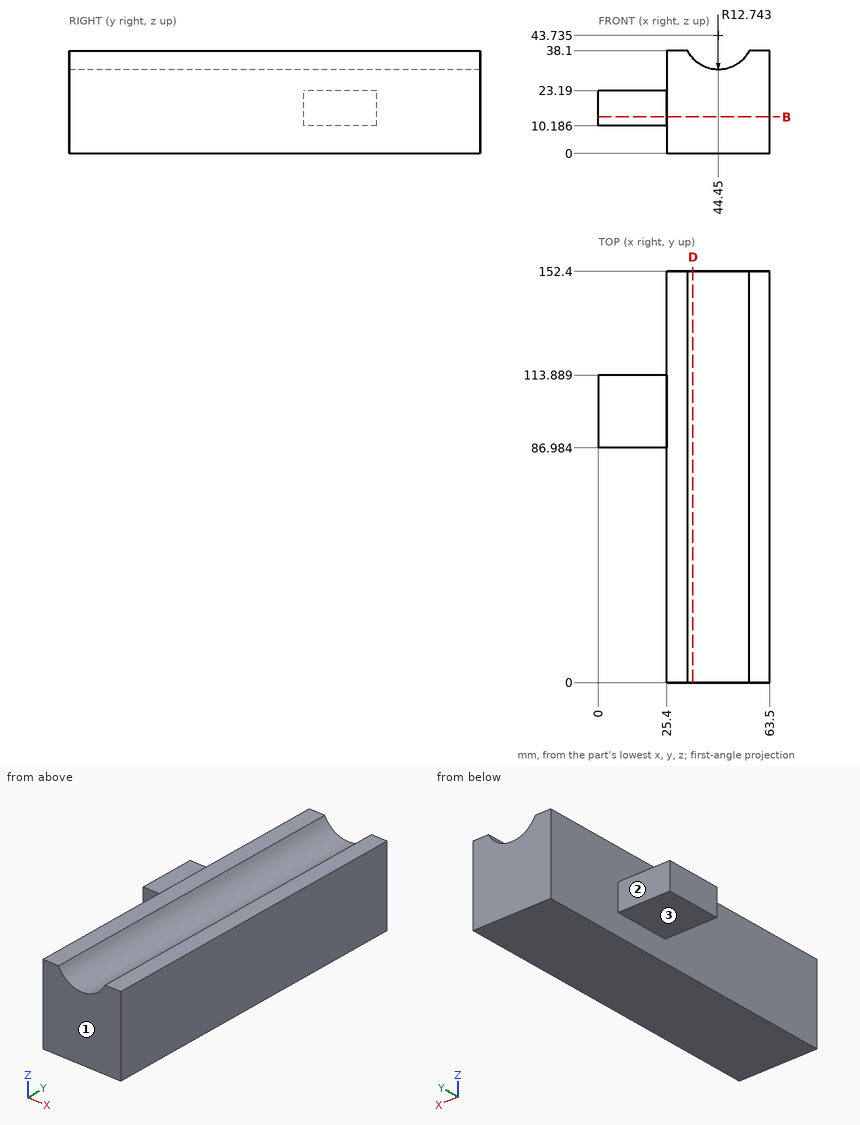
Here's the drawing with two shaded views (mm, measured from the low corner). I have some questions. A direction names the side the tool comes from. Coordinates: 2 decimals unless noted, no trailing zeros. Order: outer loops, then holes, each group sorted by start corner. A loop starts at its lowest first (then second) coordinate and runs counter-clockwise, first axis right, second up. Notation, with made-up numbers: (-3, 54.5) - (9, 54.5) arc R28 ccw to (9, 75.5) - close; hole circle Ø9 at (27.25, -5). An arc over 180 degrees is marked (long way). Answer in a Markdown table with one row per item. Add a question column.
(1) If we section it at B-B, the plane z = 13.5: Please give me the cut outline in (x, y).
(2) If we section it at D-D, the plane x = 35: Please give me the cut outline in (y, z) (1 decimal).
(3) I need wall thicknesses on L1, parallel to Y at x = 14, z = 16; L2, parallel to X at y = 134.5, z = 3; L3, parallel to X at y = 94, z = 35. Which ranges of each line are inside material? Lowest first, please.
(4) On a 3-axis mill with a long thin cutter (end or side, diameter ignored), from which of +Z, -Z, +X, -X, +Y, -Y can I reach the whole of each face in a straight line? I mean the marked faces 1, 2 and 3. Say none if no direction works.
(5) Will these pins go through, and if not, where does the flat tip stop? pin 1 (1.5 mm diameter, centred on y = 69, z = 18, fed in from -X); pin 2 (2 mm diameter, centred on x = 45.5, y = 98.5, fed in from +Z); pin 3 (6.5 mm diameter, centred on x = 12, z = 14.5, fed in from -Y).
Results are:
| question | item | result |
|---|---|---|
| 1 | outline | (0, 86.98) - (25.4, 86.98) - (25.4, 0) - (63.5, 0) - (63.5, 152.4) - (25.4, 152.4) - (25.4, 113.89) - (0, 113.89) - close |
| 2 | outline | (0, 0) - (152.4, 0) - (152.4, 35.2) - (0, 35.2) - close |
| 3 | L1 | y = 86.98 to 113.89 |
| 3 | L2 | x = 25.4 to 63.5 |
| 3 | L3 | x = 25.4 to 35.17, 53.73 to 63.5 |
| 4 | face 1 | +Z, -Z, +X, -X, -Y |
| 4 | face 2 | +Z, -Z, -X, +Y |
| 4 | face 3 | -Z, -X, +Y, -Y |
| 5 | pin 1 | stops at x = 25.4 |
| 5 | pin 2 | stops at z = 31.16 |
| 5 | pin 3 | stops at y = 86.98 |
